Build history of the part. All positions in model axes, mm. Coordinates: 2 decimals unless noted, no trailing zeros. Loops run counter-clockwise (first coordinate to the right, second up) from the corner with the lowest first, then second, coordinate; pieces in that order, holes last.
(1) Slice it at D-D (y = -20). Give the cut face in (x, z).
(2) Slice it at C-C (x = -8). Give the cut face in (y, z).
(3) Slice it at A-A (y = 0). Give the cut face in (x, z).
(4) Wall check: L1, parallel to Y at x = 0, z = 2; L2, parallel to X at y = 7, z = 1.85; L3, parallel to Y at x = -22, z = 1.9. Give the ranges that are in metal, low to high.
(5) Two-plate mould, pull along Y, no slides. Class faces 1 (the face through (-8.67, -39.05, 1.48)), 2 (the face through (9, -29, 3)), 3 (the face through (-38.29, -0.17, 1.52)): pulls with the +Y half, pulls with the -Y half, needs draft (parallel to the pull), parting line crosses it, or undercut.
(6) Flat gauge pins, fed straight in: P1, Ø4, axis at x = 0, y = -37, coming from the +Z side; P2, Ø1.5, axis at y = -4, z = 2.5, coming from the -X side; P3, Ø1, axis at x = 26.5, z = 1, coming from the +Y side. Where does each tip first touch, or does it go through?
from build123d import *

# Parameters (mm, degrees)
ESQUISSE1_R                  = 40
BOSS_EXTRU_1_DEPTH           = 3
D_GAGEMENT_M21_D             = 2.6
R_P_TITION_CIRCULAIRE1_COUNT = 4
ESQUISSE4_R                  = 30
ENL_V_MAT_EXTRU_1_DEPTH      = 10


with BuildPart() as part:
    # Esquisse1 → Boss.-Extru.1 (new body)
    with BuildSketch(Plane.XY):
        Circle(ESQUISSE1_R)
    extrude(amount=BOSS_EXTRU_1_DEPTH)

    # Dégagement M21 (through all)
    with Locations(Plane(origin=(0, 0, 0), x_dir=(-1, 0, 0), z_dir=(0, 0, -1))):
        with Locations((0, 37)):
            d_gagement_m21 = Hole(D_GAGEMENT_M21_D / 2)

    # Répétition circulaire1: Dégagement M21 ×4 about axis
    r_p_tition_circulaire1_axis = Axis((0, 0, 0), (0, 0, 1))
    for i in range(1, R_P_TITION_CIRCULAIRE1_COUNT):
        add(d_gagement_m21.rotate(r_p_tition_circulaire1_axis, i * 360 / R_P_TITION_CIRCULAIRE1_COUNT), mode=Mode.SUBTRACT)

    # Esquisse4 → Enlèv. mat.-Extru.1 (cut)
    with BuildSketch(Plane(origin=(0, 0, 0), x_dir=(-1, 0, 0), z_dir=(0, 0, -1))):
        Circle(ESQUISSE4_R)
    extrude(amount=-ENL_V_MAT_EXTRU_1_DEPTH, mode=Mode.SUBTRACT)


solid = part.part
Response values:
1. outline: (-34.64, 0) - (-22.36, 0) - (-22.36, 3) - (-34.64, 3) - close; (22.36, 0) - (34.64, 0) - (34.64, 3) - (22.36, 3) - close
2. outline: (-39.19, 0) - (-28.91, 0) - (-28.91, 3) - (-39.19, 3) - close; (28.91, 0) - (39.19, 0) - (39.19, 3) - (28.91, 3) - close
3. outline: (-40, 0) - (-38.3, 0) - (-38.3, 3) - (-40, 3) - close; (-35.7, 0) - (-30, 0) - (-30, 3) - (-35.7, 3) - close; (30, 0) - (35.7, 0) - (35.7, 3) - (30, 3) - close; (38.3, 0) - (40, 0) - (40, 3) - (38.3, 3) - close
4. L1: y = -40 to -38.3, -35.7 to -30, 30 to 35.7, 38.3 to 40
4. L2: x = -39.38 to -29.17, 29.17 to 39.38
4. L3: y = -33.41 to -20.4, 20.4 to 33.41
5. face 1: parting line crosses it
5. face 2: needs draft
5. face 3: undercut
6. P1: stops at z = 3
6. P2: stops at x = -39.87
6. P3: stops at y = 30.4
